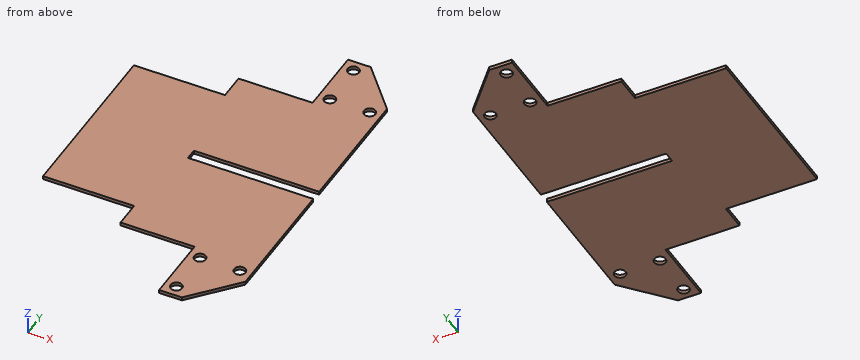
```python
from build123d import *

# Parameters (mm, degrees)
ESQUISSE1_R        = 5
BOSS_EXTRU_1_DEPTH = 3


with BuildPart() as part:
    # Esquisse1 → Boss.-Extru.1 (new body)
    with BuildSketch(Plane.XY):
        Polygon((80, 77), (0, 77), (0, 0), (90, 0), (90, 5), (200, 5), (200, 120), (165, 160), (145, 160), (145, 100), (80, 100), align=None)
        with Locations((155, 150)):
            Circle(ESQUISSE1_R, mode=Mode.SUBTRACT)
        with Locations((155, 110)):
            Circle(ESQUISSE1_R, mode=Mode.SUBTRACT)
        with Locations((190, 110)):
            Circle(ESQUISSE1_R, mode=Mode.SUBTRACT)
    boss_extru_1 = extrude(amount=BOSS_EXTRU_1_DEPTH)

    # Symétrie1: Boss.-Extru.1 across plane
    add(boss_extru_1.mirror(Plane(origin=(0, 0, 3), x_dir=(0, 0, 1), z_dir=(0, 1, 0))))


solid = part.part
```
Geometry check sheet. Reference: the model listing, model coordinates, mm. Give positions to 0.01 mm unless a question says otherwise; leave off trailing zeros. Write each loop counter-clockwise with the first axis right and the second up, starting at its lowest first coordinate (ties: lowest second). Pieces come first, ordered by that corner, then holes. Notation, with made-up numbers: (-39.75, 12.25) -> (14.25, 12.25) arc R35 cw to (14.25, 50.25) -> close; hole circle Ø3 at (21.25, 55.25). An arc over 180 degrees is marked (long way). One line per question, with ' | ' between items.
Item 1: Depth check by flat-ended pin: pin 1 (6 mm diameter, centred on x = 155, y = -150, fed in from +Z); pin 2 (1.5 mm diameter, centred on x = 118, z = 2, fed in from +Y); pin 3 (0.9 mm diameter, centred on x = 27.5, z = 1, fed in from +Y); pin 4 (1.5 mm diameter, centred on y = 118, z = 1, fed in from -X). Enter the tip coordinate at first touch or a pass-through.
Determined:
pin 1: through | pin 2: y = 100 | pin 3: y = 77 | pin 4: x = 145
Item 2: Sectioned sample at B-B, the plane x = 155. Record the boundary of the cut face in (y, z).
Determined:
outline: (-160, 0) -> (-155, 0) -> (-155, 3) -> (-160, 3) -> close; (-145, 0) -> (-115, 0) -> (-115, 3) -> (-145, 3) -> close; (-105, 0) -> (-5, 0) -> (-5, 3) -> (-105, 3) -> close; (5, 0) -> (105, 0) -> (105, 3) -> (5, 3) -> close; (115, 0) -> (145, 0) -> (145, 3) -> (115, 3) -> close; (155, 0) -> (160, 0) -> (160, 3) -> (155, 3) -> close
Item 3: Sectioned sample at A-A, the plane x = 109.5. Record the boundary of the cut face in (y, z), plus the area to 3 significant figures.
Determined:
outline: (-100, 0) -> (-5, 0) -> (-5, 3) -> (-100, 3) -> close; (5, 0) -> (100, 0) -> (100, 3) -> (5, 3) -> close | area: 570 mm^2
Item 4: Sectioned sample at D-D, the plane y = 110. Record the boundary of the cut face in (x, z).
Determined:
outline: (145, 0) -> (150, 0) -> (150, 3) -> (145, 3) -> close; (160, 0) -> (185, 0) -> (185, 3) -> (160, 3) -> close; (195, 0) -> (200, 0) -> (200, 3) -> (195, 3) -> close
Item 5: Scan lines: line 1 along Y through (x, z) = (155, 0.9); line 2 along X through (y, z) = (-110, 0.9); line 3 along Y through (x, z) = (121, 1.5). Record each from-to range of solid material in increasing order.
Determined:
line 1: -160 to -155, -145 to -115, -105 to -5, 5 to 105, 115 to 145, 155 to 160 | line 2: 145 to 150, 160 to 185, 195 to 200 | line 3: -100 to -5, 5 to 100
Item 6: Sectioned sample at C-C, the plane y = -150. Record the boundary of the cut face in (x, z), plus the area to 4 significant figures.
Determined:
outline: (145, 0) -> (150, 0) -> (150, 3) -> (145, 3) -> close; (160, 0) -> (173.75, 0) -> (173.75, 3) -> (160, 3) -> close | area: 56.25 mm^2
